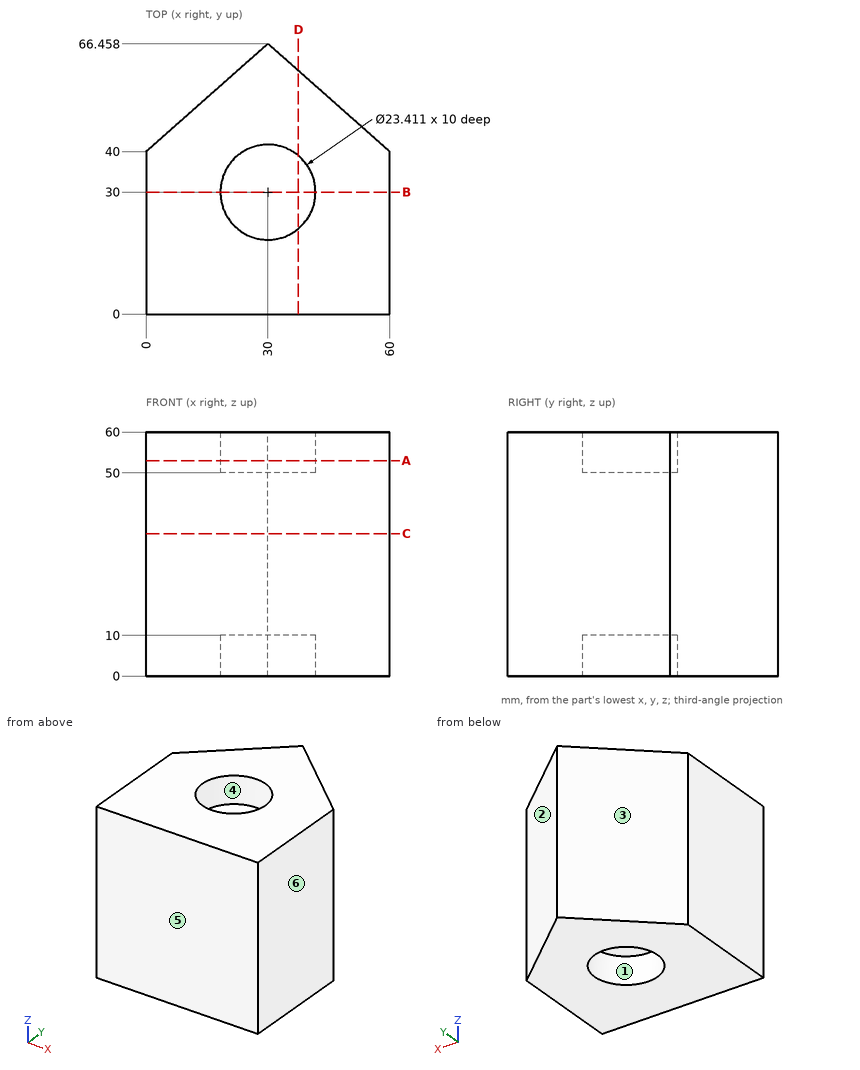
Can you work these out from the drawing? Everything is in mm from the part's minimum corner. A direction names the side the tool comes from. Round coordinates to 2 decimals unless told otherwise and drop trailing zeros. Loops run counter-clockwise (first coordinate to the right, second up) from the corner with the lowest first, then second, coordinate; pieces in that order, holes last. Notation, with made-up numbers: (61, 45.25) - (109, 45.25) arc R22 ccw to (109, 74.25) - close; hole circle Ø11 at (-7.5, 82). An arc over 180 degrees is marked (long way). One line per question, with ' | ' between items. Start each with the question number.
Q1. I want a section at B-B (y = 30). Write out the boundary of the cut face in (x, z) (1 decimal), then the cut area to 3 significant figures.
Q2. I want a section at D-D (x = 37.5). Write out the boundary of the cut face in (y, z).
Q3. I want a section at C-C (z = 35). Write out the boundary of the cut face in (x, y), then the cut area to 3 significant figures.
Q4. For the marked faces 1 and 2, which set-ups out of +Z, -Z, +X, -X, +Y, -Y let a thin tool reach every point of the face, with its end or its side?
Q5. Please list where these lines run through material, in increasing order: line 1 (Z direction, x = 30, y = 30.5); line 2 (Y direction, x = 32, z = 6.5) (1 decimal); line 3 (X direction, y = 51.5, z = 8). Write a range as [from, to].
Q6. I want a section at A-A (z = 53). Write out the boundary of the cut face in (x, y) (1 decimal), then the cut area to 3 significant figures.
Q7. Will these pins go through, and if not, where does the flat tip stop? pin 1 (2 mm diameter, centred on y = 18.5, z = 11.5, fed in from -X); pin 2 (11.5 mm diameter, centred on x = 33.5, y = 27, fed in from -Z); pin 3 (4 mm diameter, centred on y = 54, z = 44.5, fed in from -X) (1 decimal).
Q8. We'd pull the mould along X, two halves only. Please class the marked faces 3, 4, 5 and 6: +X half, -X half, draft (parallel to the pull), parting line (faces both ways), or undercut.
Response values:
1) outline: (0, 0) - (18.3, 0) - (18.3, 10) - (41.7, 10) - (41.7, 0) - (60, 0) - (60, 60) - (41.7, 60) - (41.7, 50) - (18.3, 50) - (18.3, 60) - (0, 60) - close | area: 3,130 mm²
2) outline: (0, 0) - (21.01, 0) - (21.01, 10) - (38.99, 10) - (38.99, 0) - (59.84, 0) - (59.84, 60) - (38.99, 60) - (38.99, 50) - (21.01, 50) - (21.01, 60) - (0, 60) - close
3) outline: (0, 0) - (60, 0) - (60, 40) - (30, 66.46) - (0, 40) - close | area: 3,190 mm²
4) face 1: -Z | face 2: +Z, -Z, +X, +Y
5) line 1: z = [10, 50] | line 2: y = [0, 18.5], [41.5, 64.7] | line 3: x = [13.04, 46.96]
6) outline: (0, 0) - (60, 0) - (60, 40) - (30, 66.5) - (0, 40) - close; hole circle Ø23.4 at (30, 30) | area: 2,760 mm²
7) pin 1: stops at x = 0 | pin 2: stops at z = 10 | pin 3: stops at x = 13.6
8) face 3: -X half | face 4: undercut | face 5: draft | face 6: +X half
